Could you check a few things on this model? Use its own coordinates, in mm. A direction names the side the tool comes from. Coordinates: 2 decimals unless noted, no trailing zeros. Order: outer loops, then holes, each group sorted by start corner. A loop starts at its lowest first (then second) coordinate and runs counter-clockwise, first axis right, second up. Notation, with made-up numbers: (9, -21) -> (67, -21) arc R32 ccw to (67, 9) -> close; hole circle Ø6 at (64, 35). An arc over 180 degrees is marked (long way). Return JSON: item names as keys, results as strings. Group by question number.
from build123d import *

# Parameters (mm, degrees)
F0_R     = 1.55
F1_DEPTH = 10
F3_SIZE  = 1


with BuildPart() as f1:
    # F0 (on Top) → F1 (new body)
    with BuildSketch(Plane.XY):
        with BuildLine():
            Line((16, 17.55), (0, 17.55))
            Line((0, 17.55), (0, 15.55))
            Line((0, 15.55), (16, 15.55))
            ThreePointArc((16, 15.55), (17.4142135624, 14.9642135624), (18, 13.55))
            Line((18, 13.55), (18, 7.1))
            Line((18, 7.1), (15, 7.1))
            ThreePointArc((15, 7.1), (12.4897709268, 6.0602290732), (11.45, 3.55))
            Line((11.45, 3.55), (11.45, 2))
            Line((11.45, 2), (0, 2))
            Line((0, 2), (0, 0))
            Line((0, 0), (20, 0))
            Line((20, 0), (20, 13.55))
            ThreePointArc((20, 13.55), (18.8284271247, 16.3784271247), (16, 17.55))
        make_face()
        with Locations((15, 3.55)):
            Circle(F0_R, mode=Mode.SUBTRACT)
    extrude(amount=F1_DEPTH)

    # F2: F1 across face


with BuildPart() as f1_1:
    add(f1.part)
    add(f1.part.mirror(Plane(origin=(0, 16.55, 5), x_dir=(0, -1, 0), z_dir=(-1, 0, 0))))

    # F3
    f3_edges = [f1_1.edges().sort_by_distance(p)[0] for p in [
        (-20, 0, 5),
        (20, 0, 5),
    ]]
    chamfer(f3_edges, length=F3_SIZE)


solid = f1_1.part
Q1. I want a section at D-D on y = 3. Please give me the cut outline in (x, z).
Q2. I want a section at B-B on x = 5. Please give me the cut outline in (y, z).
Q3. I'm going to push flat-ended pins straight in: pin 1 Ø8 at (x, y) = (-9.5, 15) entering from -Z; pin 2 Ø0.9 at (x, z) = (17, 5) entering from +Y; pin 3 Ø3 at (x, y) = (-2.5, 5) entering from +Z. Where does each tip first touch, or does it pass through?
Q4. On a 3-axis mill with a long thin cutter (end or side, diameter ignored), from which of +Z, -Z, +X, -X, +Y, -Y can I reach the whole of each face in a straight line? I mean faces 5 (the flat face through (18, 10, 5)), 6 (the flat face through (20, 7, 5)). Say none if no direction works.
Q5. We'd pull the mould along X, two halves only. Please class faces 1 (the flat face through (-19.5, 0.5, 4.9)), 2 (the cylindrical face through (18.859, 16.347, 4.93)), 3 (the flat face through (11.45, 3, 5)), 4 (the flat face through (0, 0, 5)): pulls with the +X half, pulls with the -X half, needs draft (parallel to the pull), parting line crosses it, or undercut.
Q6. I need wall thicknesses on line 1 along X through (y, z) = (3.5, 9); line 2 along Y through (x, z) = (-15, 2.5); line 3 along Y through (x, z) = (10, 5). Which ranges of each line are inside material? Lowest first, please. Write a range as from..to.
Q7. I want a section at C-C on z = 3.75. Please give me the cut outline in (x, y), and give its area (3 significant figures).
Q8. I want a section at A-A on y = 8.75. Please give me the cut outline in (x, z).
Response values:
{
 "1": {"outline": "(-20, 0) -> (-16.45, 0) -> (-16.45, 10) -> (-20, 10) -> close; (-13.55, 0) -> (-11.45, 0) -> (-11.45, 10) -> (-13.55, 10) -> close; (11.45, 0) -> (13.55, 0) -> (13.55, 10) -> (11.45, 10) -> close; (16.45, 0) -> (20, 0) -> (20, 10) -> (16.45, 10) -> close"},
 "2": {"outline": "(0, 0) -> (2, 0) -> (2, 10) -> (0, 10) -> close; (15.55, 0) -> (17.55, 0) -> (17.55, 10) -> (15.55, 10) -> close"},
 "3": {"pin 1": "stops at z = 0", "pin 2": "stops at y = 17.51", "pin 3": "passes through"},
 "4": {"face 5": "+Z, -Z", "face 6": "+Z, -Z, +X, +Y, -Y"},
 "5": {"face 1": "pulls with the -X half", "face 2": "pulls with the +X half", "face 3": "undercut", "face 4": "needs draft"},
 "6": {"line 1": "x = -20..-16.55, -13.45..-11.45, 11.45..13.45, 16.55..20", "line 2": "y = 0..2, 5.1..7.1, 15.55..17.55", "line 3": "y = 0..2, 15.55..17.55"},
 "7": {"outline": "(-20, 1) -> (-19, 0) -> (19, 0) -> (20, 1) -> (20, 13.55) arc R4 ccw to (16, 17.55) -> (-16, 17.55) arc R4 ccw to (-20, 13.55) -> close; hole (-18, 7.1) -> (-15, 7.1) arc R3.55 cw to (-11.45, 3.55) -> (-11.45, 2) -> (11.45, 2) -> (11.45, 3.55) arc R3.55 cw to (15, 7.1) -> (18, 7.1) -> (18, 13.55) arc R2 ccw to (16, 15.55) -> (-16, 15.55) arc R2 ccw to (-18, 13.55) -> close; hole circle Ø3.1 at (-15, 3.55); hole circle Ø3.1 at (15, 3.55)", "area": "254 mm²"},
 "8": {"outline": "(-20, 0) -> (-18, 0) -> (-18, 10) -> (-20, 10) -> close; (18, 0) -> (20, 0) -> (20, 10) -> (18, 10) -> close"}
}
